```python
from build123d import *

# Parameters (mm, degrees)
F0_R     = 11.049
F1_DEPTH = 25.4


with BuildPart() as f1:
    # F0 (on Top) → F1 (new body)
    with BuildSketch(Plane.XY):
        with BuildLine():
            ThreePointArc((9.880516, 43.696073), (10.752912, 46.100628), (11.049, 48.641354))
            ThreePointArc((11.049, 48.641354), (3.342308, 59.172706), (-9.026913, 55.012794))
            ThreePointArc((-9.026913, 55.012794), (-11.017702, 49.472403), (-9.880516, 43.696073))
            ThreePointArc((-9.880516, 43.696073), (0, 37.592354), (9.880516, 43.696073))
        make_face()
        with BuildLine():
            ThreePointArc((25.166727, 21.592547), (14.261351, 30.388211), (9.880516, 43.696073))
            ThreePointArc((9.880516, 43.696073), (0, 37.592354), (-9.880516, 43.696073))
            ThreePointArc((-9.880516, 43.696073), (-14.261351, 30.388211), (-25.166727, 21.592547))
            ThreePointArc((-25.166727, 21.592547), (-15.209211, 20.07738), (-10.618396, 11.112323))
            ThreePointArc((-10.618396, 11.112323), (-11.293541, 7.309228), (-13.236467, 3.970907))
            ThreePointArc((-13.236467, 3.970907), (-0.292561, 6.046929), (12.737323, 4.60585))
            ThreePointArc((12.737323, 4.60585), (12.750546, 17.636907), (25.166727, 21.592547))
        make_face()
        with Locations((0, 23.622)):
            Circle(F0_R, mode=Mode.SUBTRACT)
        with BuildLine():
            ThreePointArc((60.015514, 0), (45.437915, 15.390791), (25.166727, 21.592547))
            ThreePointArc((25.166727, 21.592547), (30.632453, 17.570508), (32.716396, 11.112323))
            ThreePointArc((32.716396, 11.112323), (31.227516, 5.572963), (27.162137, 1.526488))
            ThreePointArc((27.162137, 1.526488), (43.741463, 4.048326), (60.015514, 0))
        make_face()
        with BuildLine():
            ThreePointArc((32.716396, 11.112323), (30.632453, 17.570508), (25.166727, 21.592547))
            ThreePointArc((25.166727, 21.592547), (12.750546, 17.636907), (12.737323, 4.60585))
            ThreePointArc((12.737323, 4.60585), (19.360668, 0.306796), (27.162137, 1.526488))
            ThreePointArc((27.162137, 1.526488), (31.227516, 5.572963), (32.716396, 11.112323))
        make_face()
        with BuildLine():
            ThreePointArc((-10.618396, 11.112323), (-15.209211, 20.07738), (-25.166727, 21.592547))
            ThreePointArc((-25.166727, 21.592547), (-27.139076, 20.71134), (-28.902264, 19.463197))
            ThreePointArc((-28.902264, 19.463197), (-32.223312, 7.848423), (-22.92604, 0.135246))
            ThreePointArc((-22.92604, 0.135246), (-20.190383, 0.404429), (-17.484009, 0.885903))
            ThreePointArc((-17.484009, 0.885903), (-15.174357, 2.172477), (-13.236467, 3.970907))
            ThreePointArc((-13.236467, 3.970907), (-11.293541, 7.309228), (-10.618396, 11.112323))
        make_face()
        with BuildLine():
            ThreePointArc((-22.92604, 0.135246), (-32.223312, 7.848423), (-28.902264, 19.463197))
            ThreePointArc((-28.902264, 19.463197), (-45.297393, 19.057617), (-59.379004, 27.464341))
            ThreePointArc((-59.379004, 27.464341), (-46.159112, 7.121744), (-22.92604, 0.135246))
        make_face()
        with BuildLine():
            ThreePointArc((-17.484009, 0.885903), (-20.190383, 0.404429), (-22.92604, 0.135246))
            ThreePointArc((-22.92604, 0.135246), (-20.157627, 0.166959), (-17.484009, 0.885903))
        make_face()
    extrude(amount=F1_DEPTH)


solid = f1.part
```
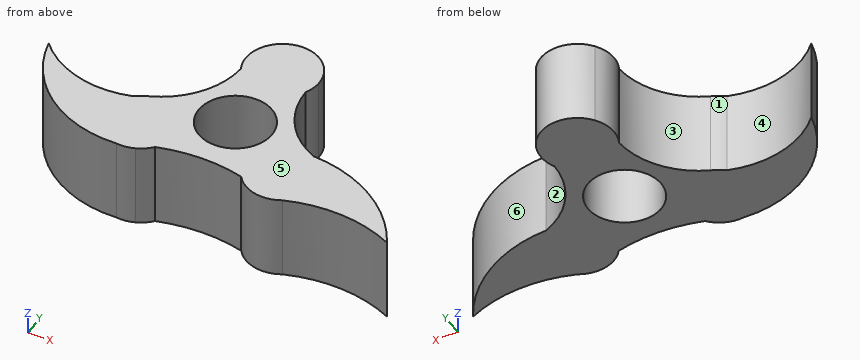
Could you check a few things on this model? Use its own coordinates, in mm. Face numbers are marked on the shaded views. A direction names the side the tool comes from. Round coordinates to 2 decimals unless told otherwise and drop trailing zeros. Loops run counter-clockwise (first coordinate to the right, second up) from the corner with the lowest first, then second, coordinate; pieces in that order, holes last.
Q1. I want a section at B-B (z = 21.5). Write out the boundary of the cut face in (x, y), and give its area (3 significant figures).
Q2. I want a section at C-C (y = 38). Write out the boundary of the cut face in (x, z), and give its area (3 significant figures).
Q3. For P1, Ø1, axis at y = 17.5, z = 11, coming from the +X side; P2, Ø12, axis at y = 29, z = 17.5, coming from the +X side; P3, Ø2, axis at y = 51.5, z = 20.5, coming from the -X side, each with a flat end and sliding along its axis, tell me the tip position at first contact or that it passes through.
Q4. On a 3-axis mill with a long thin cutter (end or side, diameter ignored), from which of +Z, -Z, +X, -X, +Y, -Y can I reach the whole of each face in a straight line? I mean the marked faces 1, 2 and 3. Say none if no direction works.
Q5. I want a section at D-D (x = -19.5). Write out the boundary of the cut face in (y, z), and give its area (3 significant figures).
Q6. Please list where these lines run through material, in increasing order: L1, parallel to X at y = 24.5, z = 12.25; L2, parallel to Y at x = 0, z = 11.75; L3, parallel to X at y = 22.5, z = 7.5.
Q7. I want a section at A-A (x = 0). Write out the boundary of the cut face in (y, z).
Q8. Thinking about a two-plate mould opening in X: for the marked faces 4, 5 and 6, which applies, pulls with the +X half, pulls with the -X half, needs draft (parallel to the pull), parting line crosses it, or undercut?
Answer below:
1. outline: (-59.38, 27.46) arc R35.26 ccw to (-22.93, 0.14) arc R11.05 ccw to (-17.48, 0.89) arc R11.05 ccw to (-13.24, 3.97) arc R48.85 cw to (12.74, 4.61) arc R11.05 ccw to (27.16, 1.53) arc R42.76 cw to (60.02, 0) arc R41.57 ccw to (25.17, 21.59) arc R24.74 cw to (9.88, 43.7) arc R11.05 ccw to (11.05, 48.64) arc R11.05 ccw to (-9.03, 55.01) arc R11.05 ccw to (-9.88, 43.7) arc R24.74 cw to (-25.17, 21.59) arc R11.05 ccw to (-28.9, 19.46) arc R29.52 cw to start; hole circle Ø22.1 at (0, 23.62)
1. area: 2,340 mm2
2. outline: (-10.73, 0) - (10.73, 0) - (10.73, 25.4) - (-10.73, 25.4) - close
2. area: 545 mm2
3. P1: stops at x = 42.6
3. P2: stops at x = 22.3
3. P3: stops at x = -10.89
4. face 1: +Z, -Z, +Y
4. face 2: +Z, -Z, +X
4. face 3: +Z, -Z
5. outline: (0.28, 0) - (24.87, 0) - (24.87, 25.4) - (0.28, 25.4) - close
5. area: 625 mm2
6. L1: x = -58.56 to -56.17, -19.99 to -11.01, 11.01 to 19.99
6. L2: y = 6.05 to 12.57, 34.67 to 59.69
6. L3: x = -57.85 to -53.32, -23.21 to -10.99, 10.99 to 23.21
7. outline: (6.05, 0) - (12.57, 0) - (12.57, 25.4) - (6.05, 25.4) - close; (34.67, 0) - (59.69, 0) - (59.69, 25.4) - (34.67, 25.4) - close
8. face 4: undercut
8. face 5: needs draft
8. face 6: pulls with the +X half
